Could you check a few things on this model? Use its own coordinates, in mm. Face numbers are marked on the shaded views. A direction names the side the tool comes from. Round coordinates to 2 decimals unless told otherwise and drop trailing zeros. Write each loop counter-clockwise with the first axis right and the second up, starting at its lowest first coordinate (ties: lowest second). Pieces come first, ordered by that corner, then holes. Notation, with made-up numbers: (19, 40) -> (37, 40) arc R18 ccw to (37, 51) -> close; hole circle Ø7 at (-39.75, 54). An arc over 180 degrees is marked (long way). Answer in a Markdown table with one row per item.
from build123d import *

# Parameters (mm, degrees)
ESQUISSE1_R             = 10
ESQUISSE1_R_2           = 5.5
BOSS_EXTRU_1_DEPTH      = 7
ESQUISSE2_R             = 6.5
ENL_V_MAT_EXTRU_1_DEPTH = 6
ESQUISSE7_W             = 12
ESQUISSE7_H             = 8
BOSS_EXTRU_2_DEPTH      = 7
CONG_1_R                = 12
TROU_TARAUD_M31_D       = 2.5
TROU_TARAUD_M51_D       = 4.2
TROU_TARAUD_M51_DEPTH   = 16
TROU_TARAUD_M51_TIP     = 1.2618073
CONG_2_R                = 1


with BuildPart() as part:
    # Esquisse1 → Boss.-Extru.1 (new body)
    with BuildSketch(Plane(origin=(0, 0, 0), x_dir=(1, 0, 0), z_dir=(0, 1, 0))):
        with Locations(Location((0, 0, 0), (0, 0, 270))):  # turned: the seam where the file's is
            Circle(ESQUISSE1_R)
        with Locations(Location((0, 0, 0), (0, 0, 270))):  # turned: the seam where the file's is
            Circle(ESQUISSE1_R_2, mode=Mode.SUBTRACT)
    extrude(amount=BOSS_EXTRU_1_DEPTH)

    # Esquisse2 → Enlèv. mat.-Extru.1 (cut)
    with BuildSketch(Plane(origin=(0, 7, 0), x_dir=(1, 0, 0), z_dir=(0, 1, 0))):
        with Locations(Location((0, 0, 0), (0, 0, 270))):  # turned: the seam where the file's is
            Circle(ESQUISSE2_R)
    extrude(amount=-ENL_V_MAT_EXTRU_1_DEPTH, mode=Mode.SUBTRACT)

    # Esquisse7 → Boss.-Extru.2 (add)
    with BuildSketch(Plane(origin=(0, 0, 0), x_dir=(1, 0, 0), z_dir=(0, 1, 0))):
        with Locations((0, -12)):
            Rectangle(ESQUISSE7_W, ESQUISSE7_H)
    extrude(amount=BOSS_EXTRU_2_DEPTH)

    # Congé1
    cong_1_edges = [part.edges().sort_by_distance(p)[0] for p in [
        (-6, 3.5, 8),
        (6, 3.5, 8),
    ]]
    fillet(cong_1_edges, radius=CONG_1_R)

    # Trou taraudé M31 (through all)
    with Locations(Plane(origin=(0, 7, 0), x_dir=(1, 0, 0), z_dir=(0, 1, 0))):
        with Locations((4.5, -7.794228634), (-4.5, -7.794228634)):
            Hole(TROU_TARAUD_M31_D / 2)

    # Trou taraudé M51
    with Locations(Plane.XY.offset(16)):
        with Locations((0, 3.5)):
            Hole(TROU_TARAUD_M51_D / 2, depth=TROU_TARAUD_M51_DEPTH)
            with Locations((0, 0, -(TROU_TARAUD_M51_DEPTH + TROU_TARAUD_M51_TIP / 2))):  # 118° drill point
                Cone(0, TROU_TARAUD_M51_D / 2, TROU_TARAUD_M51_TIP, mode=Mode.SUBTRACT)

    # Congé2
    cong_2_edges = [part.edges().sort_by_distance(p)[0] for p in [
        (-6, 3.5, 16),
        (6, 3.5, 16),
    ]]
    fillet(cong_2_edges, radius=CONG_2_R)


solid = part.part
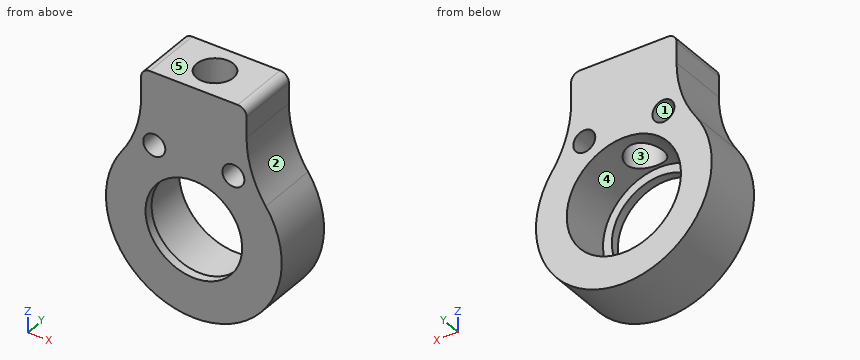
1) For pin 1 (12 mm diameter, centred on x = 6.5, z = 11, fed in from -Y); pin 2 (1.9 mm diameter, centred on y = 5, z = 13.5, fed in from +X); pin 3 (1.2 mm diameter, centred on y = 5, z = 14, fed in from -X); pin 4 (1.5 mm diameter, centred on y = 4, z = 2, fed in from +X), each with a flat end and sliding along its axis, tell me the tip position at first contact or that it passes through.
Findings:
| item | result |
|---|---|
| pin 1 | stops at y = 0 |
| pin 2 | stops at x = 6 |
| pin 3 | stops at x = -6 |
| pin 4 | stops at x = 9.92 |
2) Imagine slicing it at C-C, the plane y = 4.75. Please give me the cut outline in (x, z), plus the area to 3 significant figures.
Findings:
| item | result |
|---|---|
| outline | (-8.18, 5.75) arc R10 ccw (long way) to (8.18, 5.75) arc R12 cw to (6, 12.65) -> (6, 15) arc R1 ccw to (5, 16) -> (1.69, 16) -> (1.69, 6.28) arc R6.5 cw (long way) to (-1.69, 6.28) -> (-1.69, 16) -> (-5, 16) arc R1 ccw to (-6, 15) -> (-6, 12.65) arc R12 cw to start; hole circle Ø2.5 at (-4.5, 7.79); hole circle Ø2.5 at (4.5, 7.79) |
| area | 223 mm^2 |
3) Please list where these lines run through material, in increasing order: line 1 (X direction, y = 3.5, z = 13); line 2 (X direction, y = 0.3, z = 0); line 3 (Z direction, x = 5.25, y = 5.25).
Findings:
| item | result |
|---|---|
| line 1 | x = -6 to -2.1, 2.1 to 6 |
| line 2 | x = -10 to -5.5, 5.5 to 10 |
| line 3 | z = -8.51 to -3.83, 3.83 to 6.79, 8.79 to 15.97 |
4) Imagine slicing it at A-A, the plane z = 0. Please give me the cut outline in (x, y).
Findings:
| item | result |
|---|---|
| outline | (-10, 0) -> (-5.5, 0) -> (-5.5, 1) -> (-6.5, 1) -> (-6.5, 7) -> (-10, 7) -> close; (5.5, 0) -> (10, 0) -> (10, 7) -> (6.5, 7) -> (6.5, 1) -> (5.5, 1) -> close |
5) Imagine slicing it at D-D, the plane z = 3. Please give me the cut outline in (x, y), plus the area to 3 significant figures.
Findings:
| item | result |
|---|---|
| outline | (-9.54, 0) -> (-4.61, 0) -> (-4.61, 1) -> (-5.77, 1) -> (-5.77, 7) -> (-9.54, 7) -> close; (4.61, 0) -> (9.54, 0) -> (9.54, 7) -> (5.77, 7) -> (5.77, 1) -> (4.61, 1) -> close |
| area | 55.1 mm^2 |
6) Thinking about a two-plate mould opening in Z: for the marked faces 1, 2 and 3, which applies, +Z half, -Z half, draft (parallel to the pull), parting line (faces both ways), or undercut?
Findings:
| item | result |
|---|---|
| face 1 | undercut |
| face 2 | +Z half |
| face 3 | draft |
7) For the marked faces 4 and 5, which set-ups out of +Z, -Z, +X, -X, +Y, -Y let a thin tool reach every point of the face, with its end or its side?
Findings:
| item | result |
|---|---|
| face 4 | +Y |
| face 5 | +Z, +X, -X, +Y, -Y |
8) Imagine slicing it at B-B, the plane x = 4.5. Please give me the cut outline in (y, z).
Findings:
| item | result |
|---|---|
| outline | (0, -8.93) -> (7, -8.93) -> (7, -4.69) -> (1, -4.69) -> (1, -3.16) -> (0, -3.16) -> close; (0, 3.16) -> (1, 3.16) -> (1, 4.69) -> (7, 4.69) -> (7, 6.54) -> (0, 6.54) -> close; (0, 9.04) -> (7, 9.04) -> (7, 16) -> (0, 16) -> close |
